from build123d import *

# Parameters (mm, degrees)
CROQUIS1_W              = 20
CROQUIS1_H              = 20
SALIENTE_EXTRUIR1_DEPTH = 1
CROQUIS2_W              = 6
CROQUIS2_H              = 8
SALIENTE_EXTRUIR2_DEPTH = 1
REDONDEO1_R             = 0.2
CROQUIS3_W              = 3
CROQUIS3_H              = 3
SALIENTE_EXTRUIR3_DEPTH = 2
CROQUIS4_W              = 2
CROQUIS4_H              = 20
SALIENTE_EXTRUIR4_DEPTH = 2.5


with BuildPart() as part:
    # Croquis1 → Saliente-Extruir1 (new body)
    with BuildSketch(Plane(origin=(0, 0, 0), x_dir=(1, 0, 0), z_dir=(0, 1, 0))):
        Rectangle(CROQUIS1_W, CROQUIS1_H)
    extrude(amount=SALIENTE_EXTRUIR1_DEPTH)

    # Croquis2 → Saliente-Extruir2 (add)
    with BuildSketch(Plane(origin=(0, 1, 0), x_dir=(1, 0, 0), z_dir=(0, 1, 0))):
        with Locations((0, -1)):
            Rectangle(CROQUIS2_W, CROQUIS2_H)
    extrude(amount=SALIENTE_EXTRUIR2_DEPTH)

    # Redondeo1
    redondeo1_edges = [part.edges().sort_by_distance(p)[0] for p in [
        (3, 2, 1),
        (0, 2, -3),
        (-3, 2, 1),
        (0, 2, 5),
    ]]
    fillet(redondeo1_edges, radius=REDONDEO1_R)

    # Croquis3 → Saliente-Extruir3 (add)
    with BuildSketch(Plane(origin=(0, 1, 0), x_dir=(1, 0, 0), z_dir=(0, 1, 0))):
        with Locations((0, 6.5)):
            Rectangle(CROQUIS3_W, CROQUIS3_H)
    extrude(amount=SALIENTE_EXTRUIR3_DEPTH)

    # Croquis4 → Saliente-Extruir4 (add)
    with BuildSketch(Plane.XZ):
        with Locations((-7.5, 0)):
            Rectangle(CROQUIS4_W, CROQUIS4_H)
        with Locations((7.5, 0)):
            Rectangle(CROQUIS4_W, CROQUIS4_H)
    extrude(amount=SALIENTE_EXTRUIR4_DEPTH)


solid = part.part
Can you work these out from the model? Positions are in its coordinate system, mm. A direction names the side the tool comes from. Round coordinates to 2 decimals unless told otherwise and drop trailing zeros. Write each loop counter-clockwise with the first axis right and the second up, starting at its lowest first coordinate (ties: lowest second). Pieces come first, ordered by that corner, then holes. Notation, with made-up numbers: M 68.5,-23 L 126.5,-23 A14 cw 126.5,-17 Z; hole C 21,36 d3. An arc over 180 degrees is marked long. Use a Markdown table: item, result.
Item 1: For pin 1 Ø0.8 at (y, z) = (-1, 1.5) entering from -X; pin 2 Ø1.6 at (x, z) = (-9.5, -2.5) entering from -Y; pin 3 Ø0.8 at (y, z) = (-1.5, -0.5) entering from +X, each with a flat end and sliding along its axis, tell me the tip position at first contact or that it passes through.
Found:
| item | result |
|---|---|
| pin 1 | stops at x = -8.5 |
| pin 2 | stops at y = 0 |
| pin 3 | stops at x = 8.5 |
Item 2: I want a section at D-D (y = 1.3). List the corners of the cut face in (x, z) for me.
Found:
| item | result |
|---|---|
| outline | M -3,-3 L 3,-3 L 3,5 L -3,5 Z; M -1.5,-8 L 1.5,-8 L 1.5,-5 L -1.5,-5 Z |
Item 3: We'd pull the mould along Z, two halves only. Please class faces 6 (the face through (0, 2, -5)), 7 (the face through (-0.1, 0.4, 10)), 8 (the face through (-9, 0, 0)): released by +Z, released by -Z, zero draft, split by the parting line, or undercut.
Found:
| item | result |
|---|---|
| face 6 | undercut |
| face 7 | released by +Z |
| face 8 | zero draft |
Item 4: If I drill on line 1 along X through (y, z) = (-1.25, 2.25); line 2 along Z through (x, y) = (-1, 1.15); line 3 along X through (y, z) = (1.75, -6.75), over which ranges is the centre line in solid material (lowest first)? Write a range as [from, to].
Found:
| item | result |
|---|---|
| line 1 | x = [-8.5, -6.5], [6.5, 8.5] |
| line 2 | z = [-8, -5], [-3, 5] |
| line 3 | x = [-1.5, 1.5] |
Item 5: I want a section at C-C (z = -1.5). List the corners of the cut face in (x, y) for me, and give its area (3 significant figures).
Found:
| item | result |
|---|---|
| outline | M -10,0 L -8.5,0 L -8.5,-2.5 L -6.5,-2.5 L -6.5,0 L 6.5,0 L 6.5,-2.5 L 8.5,-2.5 L 8.5,0 L 10,0 L 10,1 L 3,1 L 3,1.8 A0.2 ccw 2.8,2 L -2.8,2 A0.2 ccw -3,1.8 L -3,1 L -10,1 Z |
| area | 36.0 mm2 |
Item 6: I want a section at B-B (x = 1). List the corners of the cut face in (y, z) for me, and give its area (3 significant figures).
Found:
| item | result |
|---|---|
| outline | M 0,-10 L 1,-10 L 1,-8 L 3,-8 L 3,-5 L 1,-5 L 1,-3 L 1.8,-3 A0.2 ccw 2,-2.8 L 2,4.8 A0.2 ccw 1.8,5 L 1,5 L 1,10 L 0,10 Z |
| area | 34.0 mm2 |
Item 7: I want a section at A-A (y = -0.55). List the corners of the cut face in (x, z) for me, and give its area (3 significant figures).
Found:
| item | result |
|---|---|
| outline | M -8.5,-10 L -6.5,-10 L -6.5,10 L -8.5,10 Z; M 6.5,-10 L 8.5,-10 L 8.5,10 L 6.5,10 Z |
| area | 80.0 mm2 |
Item 8: Which directions (+Z, -Z, +X, -X, +Y, -Y) give clear straight access to the entire face, cutting with the end or side of a thin tool? Please do faces 1 (the face through (-8.5, -1, 0)), 2 (the face through (-1.5, 2, -6)), 3 (the face through (0, 2, 1)), 4 (the face through (6.5, -1, 0)), 5 (the face through (1.5, 2, -6)).
Found:
| item | result |
|---|---|
| face 1 | +Z, -Z, -X, -Y |
| face 2 | -Z, -X, +Y |
| face 3 | +Z, +X, -X, +Y |
| face 4 | +Z, -Z, -Y |
| face 5 | -Z, +X, +Y |
